Input: part model. Units: mm. Frame: model coordinates. A direction names the side the tool comes from. Coordinates: 2 decimals unless noted, no trailing zeros. Loops run counter-clockwise (first coordinate to the right, second up) from the corner with the lowest first, then second, coordinate; pieces in that order, holes last.
Autodesk Inventor part; units mm, degrees
ref_plane "YZ Plane" through (0, 0, 0) normal (1, 0, 0) x (0, 1, 0)
ref_plane "XZ Plane" through (0, 0, 0) normal (0, 1, 0) x (-1, 0, 0)
ref_plane "XY Plane" through (0, 0, 0) normal (0, 0, 1) x (1, 0, 0)
sketch "Эскиз1" plane through (0, 0, 0) normal (0, 0, 1) x (1, 0, 0)
  line L0 (-26.5, -35) -> (13.5, -35)
  line L1 (13.5, -35) -> (13.5, 33)
  line L2 (13.5, 33) -> (-26.5, 33)
  line L3 (-26.5, 33) -> (-26.5, -35)
  line L4 (-22.5, -16.6) -> (-14.5, -16.6)
  line L5 (-14.5, -16.6) -> (-14.5, -12.6)
  line L6 (-14.5, -12.6) -> (-22.5, -12.6)
  line L7 (-22.5, -12.6) -> (-22.5, -16.6)
  line L8 (1.5, -16.6) -> (9.5, -16.6)
  line L9 (9.5, -16.6) -> (9.5, -12.6)
  line L10 (9.5, -12.6) -> (1.5, -12.6)
  line L11 (1.5, -12.6) -> (1.5, -16.6)
  line L12 (-22.5, 16.6) -> (-14.5, 16.6)
  line L13 (-14.5, 16.6) -> (-14.5, 12.6)
  line L14 (-14.5, 12.6) -> (-22.5, 12.6)
  line L15 (-22.5, 12.6) -> (-22.5, 16.6)
  line L16 (1.5, 12.6) -> (9.5, 12.6)
  line L17 (9.5, 12.6) -> (9.5, 16.6)
  line L18 (9.5, 16.6) -> (1.5, 16.6)
  line L19 (1.5, 16.6) -> (1.5, 12.6)
  line L20 (-18.5, -12.6) -> (-18.5, -3.7782) construction
  line L21 (5.5, -12.6) -> (5.5, -5.4201) construction
  point P0 (0, 0)
  point P1 (-14.5, -14.6)
  point P2 (1.5, -14.6)
  point P3 (5.5, 12.6)
  point P4 (-18.5, 12.6)
  dimension "d0" = 68
  dimension "d1" = 40
  dimension "d2" = 8
  dimension "d3" = 4
  dimension "d5" = 4
  dimension "d10" = 8
  dimension "d12" = 4
  dimension "d13" = 16
  dimension "d32" = 8
  dimension "d33" = 4
  dimension "d34" = 8
  dimension "d35" = 25.2
  dimension "d54" = 16.4
  dimension "d55" = 25.2
extrude "Выдавливание1" add sketch "Эскиз1" along normal blind 4
sketch "Эскиз3" plane through (0, 0, 4) normal (0, 0, 1) x (1, 0, 0)
  line L0 (1.5, -16.6) -> (1.5, -12.6)
  line L1 (-14.5, -12.6) -> (-14.5, -16.6)
  circle A0 centre (-6.5, 14.6) radius 1.6
  circle A1 centre (-6.5, -14.6) radius 1.6
  line L2 (-14.5, 14.6) -> (1.5, 14.6)
  line L3 (-14.5, -14.6) -> (1.5, -14.6)
  line L4 (-14.5, 16.6) -> (-14.5, 12.6)
  line L5 (1.5, 12.6) -> (1.5, 16.6)
  point P0 (0, 0)
  point P1 (-14.5, 14.6)
  point P2 (1.5, 14.6)
  dimension "d27" = 3.2
  dimension "d28" = 3.2
extrude "Выдавливание3" cut sketch "Эскиз3" against normal blind 4
sketch "Эскиз4" plane through (0, 0, 0) normal (0, 0, -1) x (-1, 0, 0)
  line L0 (-25.5, 33) -> (9.5, 33) construction
  line L1 (9.5, 33) -> (9.5, 19) construction
  line L2 (9.5, 19) -> (-25.5, 19) construction
  line L3 (-25.5, 19) -> (-25.5, 33) construction
  line L4 (-13.5, 33) -> (26.5, 33)
  line L5 (-13.5, -35) -> (-13.5, 33)
  circle A0 centre (2.5, 26) radius 1.6
  line L6 (7.5, 21) -> (7.5, 31) construction
  line L7 (8.5, 22) -> (8.5, 30)
  line L8 (6.5, 30) -> (6.5, 22)
  arc A1 (6.5, 22) -> (8.5, 22) centre (7.5, 22) ccw
  arc A2 (8.5, 30) -> (6.5, 30) centre (7.5, 30) ccw
  line L9 (9.5, 26) -> (-1.5724, 26)
  point P0 (0, 0)
  point P1 (-8, 33)
  point P2 (-25.5, 26)
  point P3 (7.5, 26)
  dimension "d39" = 35
  dimension "d40" = 14
  dimension "d41" = 12
  dimension "d42" = 3.2
  dimension "d43" = 7
  dimension "d44" = 10
  dimension "d45" = 2
  dimension "d46" = 5
extrude "Выдавливание4" cut sketch "Эскиз4" against normal blind 4
sketch "Эскиз5" plane through (0, 0, 4) normal (0, 0, 1) x (1, 0, 0)
  line L0 (4.3225, 4.75) -> (4.3225, -4.75)
  line L1 (0, 0) -> (13.5, 0) construction
  line L2 (13.5, -35) -> (13.5, 33) construction
  circle A0 centre (4.3225, 4.75) radius 1.3
  circle A1 centre (4.3225, -4.75) radius 1.3
  point P0 (4.3225, 0)
  dimension "d49" = 9.5
  dimension "d50" = 2.6
  dimension "d51" = 2.6
extrude "Выдавливание5" cut sketch "Эскиз5" against normal blind 4
sketch "Эскиз7" plane through (0, 0, 4) normal (0, 0, 1) x (1, 0, 0)
  line L0 (23.5, -19) -> (23.5, -23) construction
  line L1 (-19.8, -23) -> (-19.8, -27) construction
  line L2 (-19.8, -27) -> (-36.5, -27) construction
  line L3 (-36.5, -27) -> (-36.5, -23) construction
  line L4 (-36.5, -23) -> (-19.8, -23) construction
  line L5 (3.5, -23) -> (3.5, -27) construction
  line L6 (3.5, -27) -> (-16.5, -27) construction
  line L7 (-16.5, -27) -> (-16.5, -23) construction
  line L8 (-16.5, -23) -> (3.5, -23) construction
  line L9 (6.8, -27) -> (6.8, -23) construction
  line L10 (6.8, -23) -> (23.5, -23) construction
  line L11 (23.5, -23) -> (23.5, -27) construction
  line L12 (23.5, -27) -> (6.8, -27) construction
  line L13 (-19.8, -27) -> (-16.5, -23) construction
  line L14 (3.5, -27) -> (6.8, -23) construction
  circle A0 centre (-18.15, -25) radius 1.6
  circle A1 centre (5.15, -25) radius 1.6
  dimension "d60" = 3.2
  dimension "d61" = 3.2
extrude "Выдавливание6" cut sketch "Эскиз7" against normal blind 10
properties part number "дно_каретки"
Item 1: Section query C-C (y = 26). Output: boundary loops of the cut face in (x, z), then the cut area to 3 significant figures.
Result:
outline: (-26.5, 0) - (-8.5, 0) - (-8.5, 4) - (-26.5, 4) - close; (-6.5, 0) - (-4.1, 0) - (-4.1, 4) - (-6.5, 4) - close; (-0.9, 0) - (13.5, 0) - (13.5, 4) - (-0.9, 4) - close
area: 139 mm2
Item 2: Section query B-B (x = 8.5). Output: boundary loops of the cut face in (y, z), then the cut area to 3 significant figures.
Result:
outline: (-35, 0) - (-16.6, 0) - (-16.6, 4) - (-35, 4) - close; (-12.6, 0) - (12.6, 0) - (12.6, 4) - (-12.6, 4) - close; (16.6, 0) - (33, 0) - (33, 4) - (16.6, 4) - close
area: 240 mm2
Item 3: Reachability of faces 1 (the face through (1.5, -15, 2)), 2 (the face through (13.5, -1, 2)) from +Z, -Z, +X, -X, +Y, -Y: full face, straight path, thin tool, end or side. Return the list, or none.
Result:
face 1: +Z, -Z
face 2: +Z, -Z, +X, +Y, -Y
Item 4: Line query: L1, parallel to Y at x = -20.5, z = 3.4; L2, parallel to Y at x = -18.15, z = 1.4; L3, parallel to Y at x = -2.5, z = 1.9. Output: solid intervals per line, ascending.
Result:
L1: y = -35 to -16.6, -12.6 to 12.6, 16.6 to 33
L2: y = -35 to -26.6, -23.4 to -16.6, -12.6 to 12.6, 16.6 to 33
L3: y = -35 to 24.4, 27.6 to 33
Item 5: Section query A-A (y = -4.75). Output: boundary loops of the cut face in (x, z), then the cut area to 3 significant figures.
Result:
outline: (-26.5, 0) - (3.02, 0) - (3.02, 4) - (-26.5, 4) - close; (5.62, 0) - (13.5, 0) - (13.5, 4) - (5.62, 4) - close
area: 150 mm2
Item 6: Section query D-D (z = 0.95). Count the separate pieces of the cut face and the enclosed holes in it, then the cut area to 3 significant figures.
Result:
separate pieces: 1
enclosed holes: 12
area: 2,520 mm2
Item 7: Mould query, pull axis Y, two halves, no side actions, for faces 3 (the face through (-22.5, 15, 2)), 4 (the face through (-7, -1, 0)), 5 (the face through (-14.5, -15, 2)), 6 (the face through (-7, -35, 2)). Classes: +Y half, -Y half, draft (parallel to the pull), parting line (faces both ways), or undercut.
Result:
face 3: undercut
face 4: draft
face 5: undercut
face 6: -Y half
Item 8: Contact query for a flat-ended pin moving along its axis: P1, Ø3, axis at x = -2.5, y = 26, coming from the +Z side. Output: stop coordinate, or through.
Result:
P1: passes through
